Verification items for this drawing (mm, ordinates from the low corner). A direction names the side the tool comes from. Round coordinates to 2 decimals unless told otherwise and drop trailing zeros. Order: outer loops, then holes, each group sorted by start corner. A loop starts at its lowest first (then second) coordinate and runs counter-clockwise, first axis right, second up.
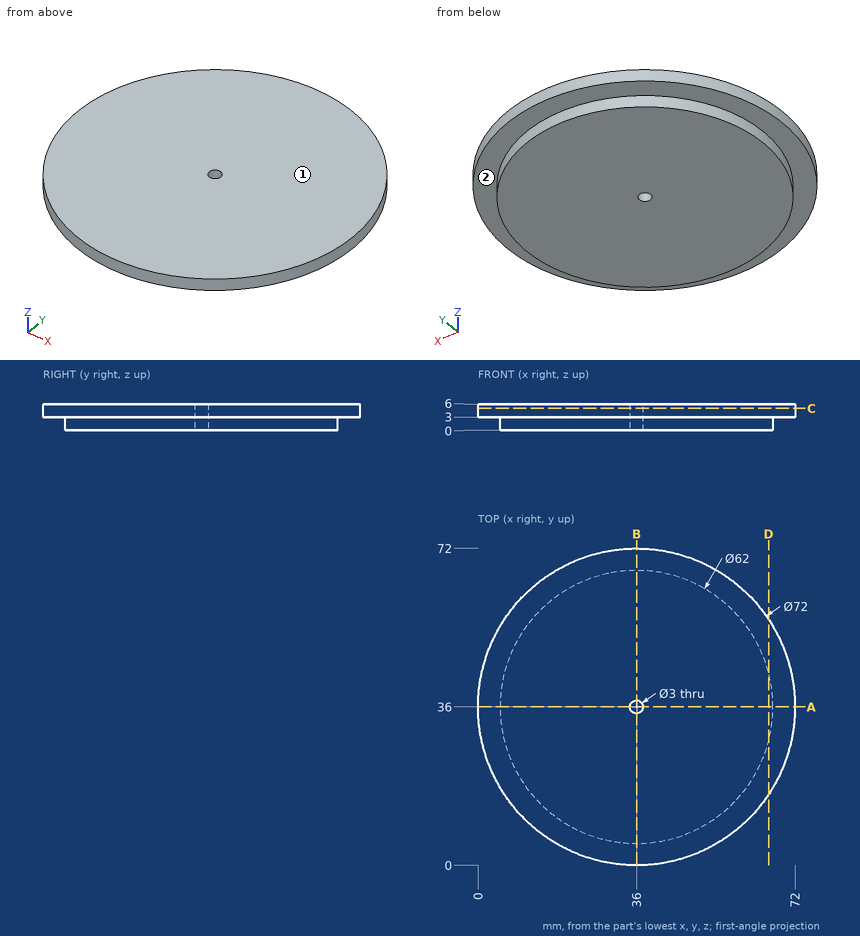
Item 1: Sectioned sample at C-C (z = 5). Record the cut outline in (x, y), and give its area (3 significant figures).
Answer:
outline: circle Ø72 at (36, 36); hole circle Ø3 at (36, 36)
area: 4,060 mm2
Item 2: Sectioned sample at A-A (y = 36). Record the cut outline in (x, z).
Answer:
outline: (0, 3) - (5, 3) - (5, 0) - (34.5, 0) - (34.5, 6) - (0, 6) - close; (37.5, 0) - (67, 0) - (67, 3) - (72, 3) - (72, 6) - (37.5, 6) - close
Item 3: Access from +Z, -Z, +X, -X, +Y, -Y to the whole of each face (thin tool, end or side, straight path). Record for the marked faces 1 and 2.
Answer:
face 1: +Z, +X, -X, +Y, -Y
face 2: -Z
Item 4: Scan lines: line 1 along Y through (x, z) = (36, 4.65); line 2 along Y through (x, z) = (36, 1.7). Record each from-to range of solid material in increasing order.
Answer:
line 1: y = 0 to 34.5, 37.5 to 72
line 2: y = 5 to 34.5, 37.5 to 67
Item 5: Sectioned sample at D-D (x = 66). Record the cut outline in (y, z), and give its area (3 significant figures).
Answer:
outline: (16.1, 3) - (28.19, 3) - (28.19, 0) - (43.81, 0) - (43.81, 3) - (55.9, 3) - (55.9, 6) - (16.1, 6) - close
area: 166 mm2
Item 6: Go/stop test with flat-tipped pins: P1, Ø1.8, axis at x = 36, y = 36, coming from the -Z side; P2, Ø3, axis at x = 62.5, z = 3.5, coming from the +Y side. Record where each tip stops, or that it passes through.
Answer:
P1: passes through
P2: stops at y = 61.9
